CAD build for the part. Positions are in the model's coordinates, mm. A direction names the side the tool comes from. Give positions to 0.01 mm unless a question says otherwise; leave off trailing zeros. Order: outer loops, then holes, each group sorted by start corner. A loop starts at its lowest first (then second) coordinate and runs counter-clockwise, first axis right, second up.
Item 1: Band-saw the part on D-D on z = -9. Give the cut face in (x, y), plus the area to 3 significant figures.
Item 2: Which spindle directions (+Z, -Z, +X, -X, +Y, -Y) get a long thin tool onto all of the face, cutting with end or side? Do faces 1 (the flat face through (20.9, -47.5, -9.8)), 2 (the flat face through (42, -50, -1)), 3 (the flat face through (0, -16, -11)), 4 (the flat face through (47, -32, -13)). Say none if no direction does.
Item 3: Band-saw the part on B-B on z = -4. Give the cut face in (x, y).
Item 4: Two-plate mould, pull along Z, no slides. Class faces 5 (the cylindrical face through (47, -16, -10)), 6 (the flat face through (0, -49, -1)), 7 (the cylindrical face through (21, -49, -13)), 8 (the flat face through (21, -28, 0)): released by +Z, released by -Z, zero draft, split by the parting line, or undercut.
Item 5: Band-saw the part on C-C on x = 21. Give the cut face in (y, z).
Item 6: Flat gauge pins, fed straight in: P1, Ø5, axis at x = -3.5, z = -15, coming from the -Y side; P2, Ø9.5, axis at x = 26.5, z = -13, coming from the +Y side; P3, Ø0.9, axis at y = -47, z = -2, coming from the +X side. Where does each tip first touch, or does it go through?
Item 7: Band-saw the part on A-A on y = -46. Give the cut face in (x, z).
Item 8: Wall check: L1, parallel to Z at x = 30, y = -17.5; L2, parallel to Y at x = 32, z = -6.25; L3, parallel to X at y = -3, z = -11. Give the ranges that are in metal, low to high.
```python
from build123d import *

# Parameters (mm, degrees)
F1_DEPTH  = 3
F0_W      = 10
F0_H      = 32
F2_DEPTH  = 13
F3_DEPTH  = 10
F4_R      = 16
F5_DEPTH  = 62.001
F6_W      = 32
F6_H      = 15
F7_DEPTH  = 23
F8_R      = 16
F9_DEPTH  = 15.001
F11_START = -3
F11_DEPTH = 4
F12_START = -55
F12_DEPTH = 4
F14_START = -5.5
F14_DEPTH = 4
F15_DEPTH = 3


with BuildPart() as f1:
    # F0 (on Top) → F1 (new body)
    with BuildSketch(Plane.XY):
        Polygon((42, 0), (0, 0), (0, -32), (0, -42), (0, -57), (42, -57), (42, -42), (42, -32), align=None)
    extrude(amount=-F1_DEPTH)

    # F0 (on Top) → F2 (join)
    with BuildSketch(Plane.XY):
        with Locations((47, -16)):
            Rectangle(F0_W, F0_H)
        with Locations((-5, -16)):
            Rectangle(F0_W, F0_H)
    extrude(amount=-F2_DEPTH)

    # F3 (add): faces of the model
    f3_faces = [f1.faces().sort_by_distance(p)[0] for p in [
        (47, -16, -13),
        (-5, -16, -13),
    ]]
    extrude(f3_faces, amount=F3_DEPTH)

    # F4 (on face) → F5 (cut, through all)
    with BuildSketch(Plane.YZ.offset(52)):
        with Locations((-16, -29)):
            Circle(F4_R)
    extrude(amount=-F5_DEPTH, mode=Mode.SUBTRACT)

    # F6 (on face) → F7 (join)
    with BuildSketch(Plane.XY):
        with Locations((21, -49.5)):
            Rectangle(F6_W, F6_H)
    extrude(amount=-F7_DEPTH)

    # F8 (on face) → F9 (cut, through all)
    with BuildSketch(Plane(origin=(0, -42, 0), x_dir=(-1, 0, 0), z_dir=(0, 1, 0))):
        with Locations((-21, -29)):
            Circle(F8_R)
    extrude(amount=-F9_DEPTH, mode=Mode.SUBTRACT)

    # F10 (on face) → F11 (cut)
    with BuildSketch(Plane(origin=(-10, 0, 0), x_dir=(0, -1, 0), z_dir=(-1, 0, 0)).offset(F11_START)):
        with BuildLine():
            ThreePointArc((0, -18.753049234), (16, -10), (32, -18.753049234))
            Line((32, -18.753049234), (32, -13.9003311295))
            ThreePointArc((32, -13.9003311295), (16, -7), (0, -13.9003311295))
            Line((0, -13.9003311295), (0, -18.753049234))
        make_face()
    extrude(amount=-F11_DEPTH, mode=Mode.SUBTRACT)

    # F10 (on face) → F12 (cut)
    with BuildSketch(Plane(origin=(-10, 0, 0), x_dir=(0, -1, 0), z_dir=(-1, 0, 0)).offset(F12_START)):
        with BuildLine():
            ThreePointArc((0, -18.753049234), (16, -10), (32, -18.753049234))
            Line((32, -18.753049234), (32, -13.9003311295))
            ThreePointArc((32, -13.9003311295), (16, -7), (0, -13.9003311295))
            Line((0, -13.9003311295), (0, -18.753049234))
        make_face()
    extrude(amount=-F12_DEPTH, mode=Mode.SUBTRACT)

    # F13 (on face) → F14 (cut)
    with BuildSketch(Plane.XZ.offset(57).offset(F14_START)):
        with BuildLine():
            ThreePointArc((5, -18.753049234), (21, -10), (37, -18.753049234))
            Line((37, -18.753049234), (37, -13.9003311295))
            ThreePointArc((37, -13.9003311295), (21, -7), (5, -13.9003311295))
            Line((5, -13.9003311295), (5, -18.753049234))
        make_face()
    extrude(amount=-F14_DEPTH, mode=Mode.SUBTRACT)

    # F0 (on Top) → F15 (join)
    with BuildSketch(Plane.XY):
        with BuildLine():
            Line((52, -32), (42, -32))
            Line((42, -32), (42, -42))
            ThreePointArc((42, -42), (44.9289321881, -34.9289321881), (52, -32))
        make_face()
        with BuildLine():
            Line((0, -42), (0, -32))
            Line((0, -32), (-10, -32))
            ThreePointArc((-10, -32), (-2.9289321881, -34.9289321881), (0, -42))
        make_face()
    extrude(amount=-F15_DEPTH)


solid = f1.part
```
The answers:
1. outline: (-10, -32) - (0, -32) - (0, 0) - (-10, 0) - close; (5, -57) - (37, -57) - (37, -42) - (5, -42) - close; (42, -32) - (52, -32) - (52, 0) - (42, 0) - close; hole (-7, -25.17) - (-3, -25.17) - (-3, -6.83) - (-7, -6.83) - close; hole (11.83, -51.5) - (30.17, -51.5) - (30.17, -47.5) - (11.83, -47.5) - close; hole (45, -25.17) - (49, -25.17) - (49, -6.83) - (45, -6.83) - close
1. area: 900 mm2
2. face 1: none
2. face 2: +Z, -Z, +X, -Y
2. face 3: -Z, +Y, -Y
2. face 4: -Z, +X, -X, -Y
3. outline: (-10, -32) - (0, -32) - (0, 0) - (-10, 0) - close; (5, -57) - (37, -57) - (37, -42) - (5, -42) - close; (42, -32) - (52, -32) - (52, 0) - (42, 0) - close
4. face 5: undercut
4. face 6: zero draft
4. face 7: released by -Z
4. face 8: released by +Z
5. outline: (-57, -13) - (-42, -13) - (-42, -3) - (0, -3) - (0, 0) - (-57, 0) - close; hole (-51.5, -10) - (-47.5, -10) - (-47.5, -7) - (-51.5, -7) - close
6. P1: stops at y = -32
6. P2: stops at y = -42
6. P3: stops at x = 42
7. outline: (0, -3) - (5, -3) - (5, -23) - (6.17, -23) arc R16 cw to (35.83, -23) - (37, -23) - (37, -3) - (42, -3) - (42, 0) - (0, 0) - close
8. L1: z = -3 to 0
8. L2: y = -57 to -42
8. L3: x = -10 to 0, 42 to 52
